Here's how the part is built. I have some questions about the finished solid (model axes, mm). A direction names the side the tool comes from. Round coordinates to 2 decimals unless told otherwise and drop trailing zeros. Loops run counter-clockwise (first coordinate to the right, second up) from the corner with the lowest first, then second, coordinate; pieces in that order, holes last. Notation, with made-up numbers: (5.25, -32.75) -> (41.25, -32.75) arc R13 cw to (41.25, -20.75) -> close; hole circle Ø8 at (-24.75, -37). An arc over 180 degrees is marked (long way). One line per item, written item: value. Start each with the question number.
```python
from build123d import *

# Parameters (mm, degrees)
F0_R     = 6
F1_DEPTH = 13.5
F3_R     = 2
F4_DEPTH = 5


with BuildPart() as f1:
    # F0 (on Top) → F1 (new body)
    with BuildSketch(Plane.XY):
        Circle(F0_R)
        with BuildLine():
            ThreePointArc((-2, 1.5), (2.5, 0), (-2, -1.5))
            Line((-2, -1.5), (-2, 1.5))
        make_face(mode=Mode.SUBTRACT)
    extrude(amount=F1_DEPTH)

    # F3 (on offset) → F4 (cut)
    with BuildSketch(Plane.YZ.offset(-6.5)):
        with Locations((0.0751335174, 6)):
            Circle(F3_R)
    extrude(amount=F4_DEPTH, mode=Mode.SUBTRACT)


solid = f1.part
```
Q1. If we mould it in two halves opening along Y, with no side actions, what happens to faces 4 (the cylindrical face through (2.5, 0.1, 6.7)), 5 (the cylindrical face through (5.723, 1.802, 6.656)), 6 (the flat face through (3, 0, 0))? For each: released by +Y, released by -Y, zero draft, split by the parting line, or undercut.
Q2. I want a section at D-D on x = -3. Please give me the cut outline in (y, z), plus the area to 3 significant figures.
Q3. I want a section at C-C on z = 9.5. Please give me the cut outline in (x, y).
Q4. If I drill on line 1 along Y through (x, z) = (0, 5); line 2 along X through (y, z) = (2, 3.75); line 3 along Y through (x, z) = (-3.8, 6), over which ranges is the centre line in solid material (lowest first)?
Q5. I want a section at B-B on y = 0. Please give me the cut outline in (x, z).
Q6. Will these pins go through, and if not, where does the flat tip stop? P1, Ø2, axis at y = -3, z = 6, coming from the +X side; P2, Ø6, axis at y = -4.5, z = 5.5, coming from the -X side; P3, Ø3, axis at y = 4, z = 8, coming from the -X side; P4, Ø3, axis at x = 0, y = 0, coming from the +Z side.
Q7. I want a section at A-A on x = 0. Please give me the cut outline in (y, z).
Q8. Which directions (+Z, -Z, +X, -X, +Y, -Y) give clear straight access to the entire face, cutting with the end or side of a thin tool? Please do faces 1 (the cylindrical face through (-3.783, 1.15, 7.686)), 2 (the flat face through (3, 0, 13.5)), 3 (the flat face through (-2, 0, 2)).
Answers below:
1. face 4: undercut
1. face 5: split by the parting line
1. face 6: zero draft
2. outline: (-5.2, 0) -> (5.2, 0) -> (5.2, 13.5) -> (-5.2, 13.5) -> close; hole circle Ø4 at (0.08, 6)
2. area: 128 mm^2
3. outline: circle Ø12 at (0, 0); hole (-2, -1.5) arc R2.5 ccw (long way) to (-2, 1.5) -> close
4. line 1: y = -6 to -2.5, 2.5 to 6
4. line 2: x = -5.66 to -1.5, 1.5 to 5.66
4. line 3: y = -4.64 to -1.92, 2.08 to 4.64
5. outline: (-6, 0) -> (-2, 0) -> (-2, 4) -> (-6, 4) -> close; (-6, 8) -> (-2, 8) -> (-2, 13.5) -> (-6, 13.5) -> close; (2.5, 0) -> (6, 0) -> (6, 13.5) -> (2.5, 13.5) -> close
6. P1: stops at x = 5.66
6. P2: stops at x = -5.79
6. P3: stops at x = -5.45
6. P4: passes through
7. outline: (-6, 0) -> (-2.5, 0) -> (-2.5, 13.5) -> (-6, 13.5) -> close; (2.5, 0) -> (6, 0) -> (6, 13.5) -> (2.5, 13.5) -> close
8. face 1: -X
8. face 2: +Z, +X, -X, +Y, -Y
8. face 3: +Z, -Z
